from build123d import *

# Parameters (mm, degrees)
BOSS_EXTRUDE1_DEPTH = 23.2
BOSS_EXTRUDE2_START = 2
SKETCH2_W           = 5
SKETCH2_H           = 1.7
BOSS_EXTRUDE2_DEPTH = 2
SKETCH3_W           = 5
SKETCH3_H           = 6
CUT_EXTRUDE1_DEPTH  = 2
SKETCH4_W           = 16.48
SKETCH4_H           = 10
CUT_EXTRUDE2_DEPTH  = 7
SKETCH6_W           = 2.8
SKETCH6_H           = 17.2
BOSS_EXTRUDE4_DEPTH = 1.3
SKETCH8_W           = 2.8
SKETCH8_H           = 17.2
BOSS_EXTRUDE5_DEPTH = 1.3
SKETCH12_W          = 12
SKETCH12_H          = 17
SKETCH12_R          = 0.95
BOSS_EXTRUDE6_DEPTH = 5
BOSS_EXTRUDE7_START = 5
SKETCH13_W          = 12
SKETCH13_H          = 17
SKETCH13_R          = 0.95
BOSS_EXTRUDE7_DEPTH = 5
CUT_EXTRUDE3_START  = -22.78
CUT_EXTRUDE3_DEPTH  = 24.78


with BuildPart() as part:
    # Sketch1 → Boss-Extrude1 (new body)
    with BuildSketch(Plane(origin=(0, 0, 0), x_dir=(1, 0, 0), z_dir=(0, 1, 0))):
        Polygon((18.223177083, -5.972057292), (-0.856822917, -5.972057292), (-0.856822917, -7.672057292), (19.923177083, -7.672057292), (19.923177083, 24.207942708), (18.223177083, 24.207942708), (18.223177083, 19.707942708), align=None)
        with BuildLine():
            Line((-0.856822917, -7.672057292), (-0.856822917, -5.972057292))
            Line((-0.856822917, -5.972057292), (-0.856822917, 19.707942708))
            Line((-0.856822917, 19.707942708), (1.966174404, 19.707942708))
            ThreePointArc((1.966174404, 19.707942708), (8.683177083, 22.792942708), (15.400179763, 19.707942708))
            Line((15.400179763, 19.707942708), (18.223177083, 19.707942708))
            Line((18.223177083, 19.707942708), (18.223177083, 24.207942708))
            Line((18.223177083, 24.207942708), (-2.556822917, 24.207942708))
            Line((-2.556822917, 24.207942708), (-2.556822917, -7.672057292))
            Line((-2.556822917, -7.672057292), (-0.856822917, -7.672057292))
        make_face()
    extrude(amount=BOSS_EXTRUDE1_DEPTH)

    # Sketch2 → Boss-Extrude2 (add)
    with BuildSketch(Plane.XZ.offset(BOSS_EXTRUDE2_START)):
        with BuildLine():
            Line((3.683177083, 5.972057292), (3.683177083, 7.672057292))
            Line((3.683177083, 7.672057292), (-2.556822917, 7.672057292))
            Line((-2.556822917, 7.672057292), (-2.556822917, -24.207942708))
            Line((-2.556822917, -24.207942708), (3.683177083, -24.207942708))
            Line((3.683177083, -24.207942708), (3.683177083, -21.246227391))
            ThreePointArc((3.683177083, -21.246227391), (2.774402431, -20.533199118), (1.966174404, -19.707942708))
            Line((1.966174404, -19.707942708), (-0.856822917, -19.707942708))
            Line((-0.856822917, -19.707942708), (-0.856822917, 5.972057292))
            Line((-0.856822917, 5.972057292), (3.683177083, 5.972057292))
        make_face()
        with BuildLine():
            Line((8.683177083, -24.207942708), (8.683177083, -22.792942708))
            ThreePointArc((8.683177083, -22.792942708), (6.066293045, -22.397431046), (3.683177083, -21.246227391))
            Line((3.683177083, -21.246227391), (3.683177083, -24.207942708))
            Line((3.683177083, -24.207942708), (8.683177083, -24.207942708))
        make_face()
        with BuildLine():
            ThreePointArc((13.683177083, -21.246227391), (11.300061121, -22.397431046), (8.683177083, -22.792942708))
            Line((8.683177083, -22.792942708), (8.683177083, -24.207942708))
            Line((8.683177083, -24.207942708), (13.683177083, -24.207942708))
            Line((13.683177083, -24.207942708), (13.683177083, -21.246227391))
        make_face()
        with BuildLine():
            Line((19.923177083, 7.672057292), (13.683177083, 7.672057292))
            Line((13.683177083, 7.672057292), (13.683177083, 5.972057292))
            Line((13.683177083, 5.972057292), (18.223177083, 5.972057292))
            Line((18.223177083, 5.972057292), (18.223177083, -19.707942708))
            Line((18.223177083, -19.707942708), (15.400179763, -19.707942708))
            ThreePointArc((15.400179763, -19.707942708), (14.591951736, -20.533199118), (13.683177083, -21.246227391))
            Line((13.683177083, -21.246227391), (13.683177083, -24.207942708))
            Line((13.683177083, -24.207942708), (19.923177083, -24.207942708))
            Line((19.923177083, -24.207942708), (19.923177083, 7.672057292))
        make_face()
        with Locations((11.183177083, 6.822057292)):
            Rectangle(SKETCH2_W, SKETCH2_H)
        with Locations((6.183177083, 6.822057292)):
            Rectangle(SKETCH2_W, SKETCH2_H)
        with BuildLine():
            Line((13.683177083, 5.972057292), (8.683177083, 5.972057292))
            Line((8.683177083, 5.972057292), (8.683177083, -22.792942708))
            ThreePointArc((8.683177083, -22.792942708), (11.300061121, -22.397431046), (13.683177083, -21.246227391))
            Line((13.683177083, -21.246227391), (13.683177083, 5.972057292))
        make_face()
        with BuildLine():
            Line((8.683177083, -22.792942708), (8.683177083, 5.972057292))
            Line((8.683177083, 5.972057292), (3.683177083, 5.972057292))
            Line((3.683177083, 5.972057292), (3.683177083, -21.246227391))
            ThreePointArc((3.683177083, -21.246227391), (6.066293045, -22.397431046), (8.683177083, -22.792942708))
        make_face()
    extrude(amount=-BOSS_EXTRUDE2_DEPTH)

    # Sketch3 → Cut-Extrude1 (cut)
    with BuildSketch(Plane.XY.offset(7.672057292)):
        with Locations((1.943177083, 15.7)):
            Rectangle(SKETCH3_W, SKETCH3_H)
    extrude(amount=-CUT_EXTRUDE1_DEPTH, mode=Mode.SUBTRACT)

    # Sketch4 → Cut-Extrude2 (cut)
    with BuildSketch(Plane(origin=(0, 0, -24.207942708), x_dir=(-1, 0, 0), z_dir=(0, 0, -1))):
        with Locations((-8.683177083, 15.2)):
            Rectangle(SKETCH4_W, SKETCH4_H)
    extrude(amount=-CUT_EXTRUDE2_DEPTH, mode=Mode.SUBTRACT)

    # Sketch6 → Boss-Extrude4 (add)
    with BuildSketch(Plane.ZY.offset(-18.223177083)):
        with Locations((-18.307942708, 6.6)):
            Rectangle(SKETCH6_W, SKETCH6_H)
    extrude(amount=BOSS_EXTRUDE4_DEPTH)

    # Sketch8 → Boss-Extrude5 (add)
    with BuildSketch(Plane(origin=(-0.856822917, 0, 0), x_dir=(0, 0, -1), z_dir=(1, 0, 0))):
        with Locations((18.307942708, 6.6)):
            Rectangle(SKETCH8_W, SKETCH8_H)
    extrude(amount=BOSS_EXTRUDE5_DEPTH)

    # Sketch12 → Boss-Extrude6 (add)
    with BuildSketch(Plane(origin=(19.923177083, 0, 0), x_dir=(0, 0, -1), z_dir=(1, 0, 0))):
        with Locations((14.267942708, 6.5)):
            Rectangle(SKETCH12_W, SKETCH12_H)
        with Locations((14.267942708, 9)):
            Circle(SKETCH12_R, mode=Mode.SUBTRACT)
    extrude(amount=BOSS_EXTRUDE6_DEPTH)

    # Sketch13 → Boss-Extrude7 (add)
    with BuildSketch(Plane.ZY.offset(2.556822917).offset(BOSS_EXTRUDE7_START)):
        with Locations((-14.267942708, 6.5)):
            Rectangle(SKETCH13_W, SKETCH13_H)
        with Locations(Location((-14.267942708, 9, 0), (0, 0, 180))):
            Circle(SKETCH13_R, mode=Mode.SUBTRACT)
    extrude(amount=-BOSS_EXTRUDE7_DEPTH)

    # Sketch15 → Cut-Extrude3 (cut)
    with BuildSketch(Plane(origin=(19.923177083, 0, 0), x_dir=(0, 0, -1), z_dir=(1, 0, 0)).offset(CUT_EXTRUDE3_START)):
        Polygon((16.773642877, 9), (15.520792792, 11.17), (13.015092624, 11.17), (11.76224254, 9), (13.015092624, 6.83), (15.520792792, 6.83), align=None)
    extrude(amount=CUT_EXTRUDE3_DEPTH, mode=Mode.SUBTRACT)


solid = part.part
Build history of the part. All positions in model axes, mm. A direction names the side the tool comes from. Coordinates: 2 decimals unless noted, no trailing zeros. Order: outer loops, then holes, each group sorted by start corner. A loop starts at its lowest first (then second) coordinate and runs counter-clockwise, first axis right, second up. Notation, with made-up numbers: M 48,34.25 L 88,34.25 A22 ccw 88,59.25 Z; hole C 86.25,25.5 d5. An arc over 180 degrees is marked long. One line per question, with ' | ' between items. Start each with the question number.
Q1. Probe L1, parallel to X at y = 9.25, z = -0.5; L2, parallel to Z at x = -4.95, y = 9; L3, parallel to Z at x = 17, y = 1.5. List the from-to ranges inside material, lowest first. Write a range as from..to.
Q2. Saw through at A-A (y = 17.25). List the corners of the cut face in (x, z), then the cut area to 3 significant figures.
Q3. Saw through at B-B (z = -18.5). List the corners of the cut face in (x, y), then the cut area to 3 significant figures.
Q4. Two-plate mould, pull along X, no slides. Class faces 4 (the face through (24.923, 7, -14)), 5 (the face through (-1.4, 23.2, -10.7)), 6 (the face through (0, 15.2, -18)): +X half, -X half, draft (parallel to the pull), parting line (faces both ways), or undercut.
Q5. Saw through at D-D (y = 1.25). List the corners of the cut face in (x, z) (3 decimals).
Q6. 3-axis set-ups, long thin cutter, end or side, ignore diameter. For faces 1 (the face through (3.683, -1, -7)), 2 (the face through (16.923, 12, -20)), 3 (the face through (18, 15.2, -18)): which of +Z, -Z, +X, -X, +Y, -Y reach the whole face in a straight line?
Q7. Saw through at C-C (x = 2.5). List the corners of the cut face in (y, z).
Q8. Flat gauge pins, fed straight in: pin 1 Ø5.5 at (x, z) = (-6, -16) entering from +Y; pin 2 Ø6 at (y, z) = (4, 3) entering from -X; pin 3 Ø4 at (x, y) = (-6, 10) entering from -Z. Where does each tip first touch, or does it go through?
Check values:
1) L1: x = -2.56..-0.86, 18.22..19.92 | L2: z = -20.27..-15.22, -13.32..-8.27 | L3: z = -24.21..-16.91, 5.97..7.67
2) outline: M -2.56,-24.21 L 0.44,-24.21 L 0.44,-19.71 L -0.86,-19.71 L -0.86,5.97 L -0.56,5.97 L -0.56,7.67 L -2.56,7.67 Z; M 4.44,5.97 L 18.22,5.97 L 18.22,-19.71 L 16.92,-19.71 L 16.92,-24.21 L 19.92,-24.21 L 19.92,7.67 L 4.44,7.67 Z | area: 144 mm2
3) outline: M -7.56,-2 L 0.44,-2 L 0.44,15.2 L -0.86,15.2 L -0.86,23.2 L -2.56,23.2 L -2.56,15 L -7.56,15 Z; M 3.68,-2 L 13.68,-2 L 13.68,0 L 3.68,0 Z; M 16.92,-2 L 24.92,-2 L 24.92,15 L 19.92,15 L 19.92,23.2 L 18.22,23.2 L 18.22,15.2 L 16.92,15.2 Z | area: 320 mm2
4) face 4: +X half | face 5: draft | face 6: undercut
5) outline: M -7.557,-20.268 L -2.557,-20.268 L -2.557,-24.208 L 19.923,-24.208 L 19.923,-20.268 L 24.923,-20.268 L 24.923,-8.268 L 19.923,-8.268 L 19.923,7.672 L -2.557,7.672 L -2.557,-8.268 L -7.557,-8.268 Z; hole M -0.857,-16.908 L 0.443,-16.908 L 0.443,-19.708 L 1.966,-19.708 A8.855 ccw 15.4,-19.708 L 16.923,-19.708 L 16.923,-16.908 L 18.223,-16.908 L 18.223,5.972 L -0.857,5.972 Z
6) face 1: +Y, -Y | face 2: none | face 3: +Y
7) outline: M -2,-24.21 L 10.2,-24.21 L 10.2,-20.28 L -2,-20.28 Z; M -2,5.97 L 12.7,5.97 L 12.7,7.67 L -2,7.67 Z; M 18.7,5.97 L 23.2,5.97 L 23.2,7.67 L 18.7,7.67 Z; M 20.2,-24.21 L 23.2,-24.21 L 23.2,-20.28 L 20.2,-20.28 Z
8) pin 1: stops at y = 15 | pin 2: stops at x = -2.56 | pin 3: stops at z = -20.27
